Can you work these out from the model? Positions are in its coordinate system, mm. A direction names the side the tool comes from. Round coordinates to 2 decimals unless told otherwise and drop trailing zeros. Order: outer loops, then holes, each group sorted by start corner. A loop starts at its lowest first (then second) coordinate and runs counter-clockwise, first axis right, second up. Notation, with made-up numbers: (29.5, -3.5) - (79.5, -3.5) arc R30 cw to (79.5, 22.5) - close; hole circle Ø8 at (64.25, 66.25). An arc over 180 degrees is marked (long way). Write item = value, one per line.
from build123d import *

# Parameters (mm, degrees)
SKETCH2_W           = 40
SKETCH2_H           = 90
BOSS_EXTRUDE1_DEPTH = 30
SKETCH3_R           = 4
CUT_EXTRUDE1_DEPTH  = 20
SKETCH4_R           = 4
SKETCH4_R_2         = 2.5
SKETCH4_W           = 3
SKETCH4_H           = 12
CUT_EXTRUDE2_DEPTH  = 10
FILLET1_R           = 10


with BuildPart() as part:
    # Sketch2 → Boss-Extrude1 (new body)
    with BuildSketch(Plane(origin=(0, 0, 0), x_dir=(1, 0, 0), z_dir=(0, 1, 0))):
        with Locations((-3.52238806, 4.76119403)):
            Rectangle(SKETCH2_W, SKETCH2_H)
    extrude(amount=BOSS_EXTRUDE1_DEPTH)

    # Sketch3 → Cut-Extrude1 (cut)
    with BuildSketch(Plane(origin=(0, 30, 0), x_dir=(1, 0, 0), z_dir=(0, 1, 0))):
        with Locations((-3.52238806, 37.26119403)):
            Circle(SKETCH3_R)
        with Locations((-3.52238806, -27.73880597)):
            Circle(SKETCH3_R)
    extrude(amount=-CUT_EXTRUDE1_DEPTH, mode=Mode.SUBTRACT)

    # Sketch4 → Cut-Extrude2 (cut)
    with BuildSketch(Plane.ZY.offset(23.52238806)):
        with Locations((2.73880597, 15)):
            Circle(SKETCH4_R)
        with Locations((2.73880597, 15)):
            Circle(SKETCH4_R_2, mode=Mode.SUBTRACT)
        with Locations((2.73880597, 24)):
            Rectangle(SKETCH4_W, SKETCH4_H)
    extrude(amount=-CUT_EXTRUDE2_DEPTH, mode=Mode.SUBTRACT)

    # Fillet1
    fillet1_edges = [part.edges().sort_by_distance(p)[0] for p in [
        (-23.52238806, 15, -49.76119403),
        (16.47761194, 15, -49.76119403),
        (16.47761194, 15, 40.23880597),
        (-23.52238806, 15, 40.23880597),
    ]]
    fillet(fillet1_edges, radius=FILLET1_R)


solid = part.part
(1) If we section it at A-A (x = -17.5): Write out the boundary of the cut face in (y, z), plus the area to 3 significant figures.
Computed:
outline = (0, -48.94) - (30, -48.94) - (30, 1.24) - (18.71, 1.24) arc R4 cw (long way) to (18.71, 4.24) - (30, 4.24) - (30, 39.41) - (0, 39.41) - close; circle Ø5 at (15, 2.74)
area = 2,590 mm^2
(2) On a 3-axis mill with a long thin cutter (end or side, diameter ignored), from which of +Z, -Z, +X, -X, +Y, -Y can I reach the whole of each face in a straight line? I mean faces 1 (the face through (-13.522, 19, 3)), 2 (the face through (-4, 10, -37)), 3 (the face through (-23.522, 15, -4)), 4 (the face through (-19, 24, 1.239)). Say none if no direction works.
Computed:
face_1 = -X
face_2 = +Y
face_3 = +Z, -Z, -X, +Y, -Y
face_4 = -X, +Y
(3) Thinking about a two-plate mould opening in X: for faces 5 (the face through (-19, 24, 4.239)), 6 (the face through (-20.671, 15.21, -46.754)), 7 (the face through (16.478, 15, -4)), 8 (the face through (-4, 10, 28)), which applies, +X half, -X half, draft (parallel to the pull), parting line (faces both ways), or undercut?
Computed:
face_5 = draft
face_6 = -X half
face_7 = +X half
face_8 = undercut
(4) If we section it at D-D (x = 13.5): Write out the boundary of the cut face in (y, z), plus the area to 3 significant figures.
Computed:
outline = (0, -46.88) - (30, -46.88) - (30, 37.36) - (0, 37.36) - close
area = 2,530 mm^2
(5) If I drill on line 1 (Z direction, x = -14.5, y = 26); line 2 (Z direction, x = -18, y = 18.5); line 3 (X direction, y = 17.75, z = -34), over which ranges is the centre line in solid material (lowest first)? Write a range as from..to.
Computed:
line_1 = -49.71..1.24, 4.24..40.19
line_2 = -48.7..0.8, 4.68..39.18
line_3 = -23.52..-5.84, -1.21..16.48
(6) Will these pins go through, and if not, where does the flat tip stop? P1, Ø3, axis at x = -20, y = 25, coming from the +Z side; P2, Ø2.5, axis at x = -2.5, z = -36.5, coming from the +Y side; P3, Ø5, axis at x = -17.5, y = 25, coming from the -Z side.
Computed:
P1 = 38.91
P2 = 10
P3 = -49.65
(7) If we section it at B-B (y = 7.25): Write out the boundary of the cut face in (x, z), plus the area to 3 significant figures.
Computed:
outline = (-23.52, -39.76) arc R10 ccw to (-13.52, -49.76) - (6.48, -49.76) arc R10 ccw to (16.48, -39.76) - (16.48, 30.24) arc R10 ccw to (6.48, 40.24) - (-13.52, 40.24) arc R10 ccw to (-23.52, 30.24) - close
area = 3,510 mm^2
(8) If we section it at C-C (y = 15): Write out the boundary of the cut face in (x, z), plus the area to 3 significant figures.
Computed:
outline = (-23.52, -39.76) arc R10 ccw to (-13.52, -49.76) - (6.48, -49.76) arc R10 ccw to (16.48, -39.76) - (16.48, 30.24) arc R10 ccw to (6.48, 40.24) - (-13.52, 40.24) arc R10 ccw to (-23.52, 30.24) - (-23.52, 6.74) - (-13.52, 6.74) - (-13.52, 5.24) - (-23.52, 5.24) - (-23.52, 0.24) - (-13.52, 0.24) - (-13.52, -1.26) - (-23.52, -1.26) - close; hole circle Ø8 at (-3.52, -37.26); hole circle Ø8 at (-3.52, 27.74)
area = 3,380 mm^2
